Here's how the part is built. I have some questions about the finished solid (model axes, mm). Face numbers are marked on the shaded views. A direction names the side the tool comes from. Round coordinates to 2 decimals unless told otherwise and drop trailing zeros. Order: outer loops, then holes, each group sorted by start corner. A loop starts at its lowest first (then second) coordinate and runs counter-clockwise, first axis right, second up. Notation, with made-up numbers: (86, 52) -> (102, 52) arc R10 cw to (102, 63) -> close; hole circle Ø8 at (-35.75, 70.25). An arc over 180 degrees is marked (long way). Use a Markdown table: item, result. Add a question column.
(1) I want a section at B-B, the plane y = 23.5. Please give me the cut outline in (x, z).
(2) On a 3-axis mill with a long thin cutter (end or side, diameter ignored), from which of +Z, -Z, +X, -X, +Y, -Y can I reach the whole of each face in a straight line? I mean the marked faces 1, 2 and 3. Say none if no direction works.
(3) I'm going to push flat-ended pins straight in: P1, Ø2.5, axis at x = 0, z = -8, coming from the +Y side; P2, Ø2, axis at x = 7, z = -7, coming from the -Y side; P3, Ø2, axis at y = 16.5, z = 3.5, coming from the +X side. Where does each tip first touch, or does it pass through?
(4) I want a section at A-A, the plane x = -1. Give the number of separate pieces and of enclosed holes in the cut face, then the cut area to 3 significant figures.
(5) Thinking about a two-plate mould opening in Y: for the marked faces 4, 5, 6 and 7, which applies, pulls with the +Y half, pulls with the -Y half, needs draft (parallel to the pull), parting line crosses it, or undercut?
(6) If I drill on probe 1 along X at (y, z) = (1.7, 0); probe 2 along Z at (x, y) = (8, 1.2), over which ranges is the centre line in solid material (lowest first)?
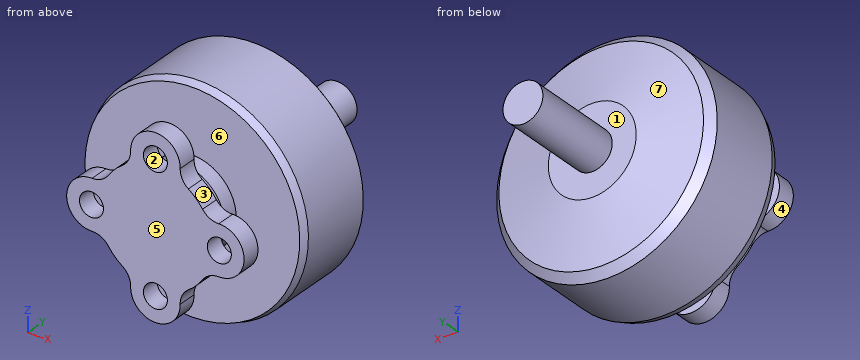
from build123d import *

# Parameters (mm, degrees)
SKETCH2_R          = 12
SKETCH2_R_2        = 1.5
CUT_EXTRUDE1_DEPTH = 35.996892719


with BuildPart() as part:
    # Sketch1 → Revolve1 (revolve)
    with BuildSketch(Plane(origin=(0, 0, 0), x_dir=(0, 0, -1), z_dir=(1, 0, 0)), mode=Mode.PRIVATE) as revolve1_sk:
        with BuildLine():
            Line((0, 0), (0, 31.45))
            Line((0, 31.45), (-2.5, 31.45))
            Line((-2.5, 31.45), (-2.5, 19.45))
            Line((-2.5, 19.45), (-5.5, 19.45))
            Line((-5.5, 19.45), (-12.8, 17.8983371))
            Line((-12.8, 17.8983371), (-13.8, 16.8983371))
            Line((-13.8, 16.8983371), (-13.8, 7.4))
            Line((-13.8, 7.4), (-13.436029766, 6.4))
            Line((-13.436029766, 6.4), (-5.5, 6.4))
            Line((-5.5, 6.4), (-5.5, 4.4))
            ThreePointArc((-5.5, 4.4), (-5.763932023, 3.281966011), (-6.5, 2.4))
            Line((-6.5, 2.4), (-12, 2.4))
            Line((-12, 2.4), (-12, 0))
            Line((-12, 0), (0, 0))
        make_face()
    revolve(revolve1_sk.sketch.rotate(Axis((0, 0, 0), (0, 1, 0)), 180), axis=Axis((0, 0, 0), (0, 1, 0)))

    # Sketch2 → Cut-Extrude1 (cut, through all)
    # profile 1 of 5: a face of its own
    with BuildSketch(Plane(origin=(0, 2.4, 0), x_dir=(1, 0, 0), z_dir=(0, 1, 0))):
        Circle(SKETCH2_R)
        with BuildLine():
            ThreePointArc((-3.09912558, -7.926375), (0, -11.1), (3.09912558, -7.926375))
            ThreePointArc((3.09912558, -7.926375), (3.357154936, -6.785464761), (4.123836457, -5.90203125))
            ThreePointArc((4.123836457, -5.90203125), (5.091168825, -5.091168825), (5.90203125, -4.123836457))
            ThreePointArc((5.90203125, -4.123836457), (6.785464761, -3.357154936), (7.926375, -3.09912558))
            ThreePointArc((7.926375, -3.09912558), (11.1, 0), (7.926375, 3.09912558))
            ThreePointArc((7.926375, 3.09912558), (6.785464761, 3.357154936), (5.90203125, 4.123836457))
            ThreePointArc((5.90203125, 4.123836457), (5.091168825, 5.091168825), (4.123836457, 5.90203125))
            ThreePointArc((4.123836457, 5.90203125), (3.357154936, 6.785464761), (3.09912558, 7.926375))
            ThreePointArc((3.09912558, 7.926375), (0, 11.1), (-3.09912558, 7.926375))
            ThreePointArc((-3.09912558, 7.926375), (-3.357154936, 6.785464761), (-4.123836457, 5.90203125))
            ThreePointArc((-4.123836457, 5.90203125), (-5.091168825, 5.091168825), (-5.90203125, 4.123836457))
            ThreePointArc((-5.90203125, 4.123836457), (-6.785464761, 3.357154936), (-7.926375, 3.09912558))
            ThreePointArc((-7.926375, 3.09912558), (-11.1, 0), (-7.926375, -3.09912558))
            ThreePointArc((-7.926375, -3.09912558), (-6.785464761, -3.357154936), (-5.90203125, -4.123836457))
            ThreePointArc((-5.90203125, -4.123836457), (-5.091168825, -5.091168825), (-4.123836457, -5.90203125))
            ThreePointArc((-4.123836457, -5.90203125), (-3.357154936, -6.785464761), (-3.09912558, -7.926375))
        make_face(mode=Mode.SUBTRACT)
    # profile 2 of 5: a face of its own
    with BuildSketch(Plane(origin=(0, 2.4, 0), x_dir=(1, 0, 0), z_dir=(0, 1, 0))):
        with Locations(Location((0, -8, 0), (0, 0, 270))):
            Circle(SKETCH2_R_2)
    # profile 3 of 5: a face of its own
    with BuildSketch(Plane(origin=(0, 2.4, 0), x_dir=(1, 0, 0), z_dir=(0, 1, 0))):
        with Locations(Location((8, 0, 0), (0, 0, 270))):
            Circle(SKETCH2_R_2)
    # profile 4 of 5: a face of its own
    with BuildSketch(Plane(origin=(0, 2.4, 0), x_dir=(1, 0, 0), z_dir=(0, 1, 0))):
        with Locations(Location((0, 8, 0), (0, 0, 270))):
            Circle(SKETCH2_R_2)
    # profile 5 of 5: a face of its own
    with BuildSketch(Plane(origin=(0, 2.4, 0), x_dir=(1, 0, 0), z_dir=(0, 1, 0))):
        with Locations(Location((-8, 0, 0), (0, 0, 270))):
            Circle(SKETCH2_R_2)
    extrude(amount=-CUT_EXTRUDE1_DEPTH, mode=Mode.SUBTRACT)


solid = part.part
Taken from the geometry:
| question | item | result |
|---|---|---|
| 1 | outline | circle Ø5 at (0, 0) |
| 2 | face 1 | +Y |
| 2 | face 2 | -Y |
| 2 | face 3 | +Z, +X, -Y |
| 3 | P1 | stops at y = 19.18 |
| 3 | P2 | stops at y = 6.4 |
| 3 | P3 | stops at x = 13.57 |
| 4 | separate pieces | 3 |
| 4 | enclosed holes | 0 |
| 4 | area | 485 mm2 |
| 5 | face 4 | needs draft |
| 5 | face 5 | pulls with the -Y half |
| 5 | face 6 | undercut |
| 5 | face 7 | pulls with the +Y half |
| 6 | probe 1 | x = -11.1 to -9.5, -6.5 to 6.5, 9.5 to 11.1 |
| 6 | probe 2 | z = -3.1 to -1.5, 1.5 to 3.1 |
